Geometry: final body of the model. Coordinates: model frame, mm. A direction names the side the tool comes from. Give positions to 0.01 mm unless a question says otherwise; leave off trailing zeros. Write each loop counter-clockwise with the first axis right and the second up, starting at its lowest first coordinate (ties: lowest second). Pieces come first, ordered by that corner, then holes.
from build123d import *

# Parameters (mm, degrees)
F1_DEPTH = 580
F2_R     = 6.25
F3_DEPTH = 80.001


with BuildPart() as f1:
    # F0 (on Front) → F1 (new body, symmetric)
    with BuildSketch(Plane.XZ):
        with BuildLine():
            ThreePointArc((40, 30), (37.071068, 37.071068), (30, 40))
            Line((30, 40), (-30, 40))
            ThreePointArc((-30, 40), (-37.071068, 37.071068), (-40, 30))
            Line((-40, 30), (-40, -30))
            ThreePointArc((-40, -30), (-37.071068, -37.071068), (-30, -40))
            Line((-30, -40), (30, -40))
            ThreePointArc((30, -40), (37.071068, -37.071068), (40, -30))
            Line((40, -30), (40, 30))
        make_face()
        with BuildLine():
            ThreePointArc((30, 35), (33.535534, 33.535534), (35, 30))
            Line((35, 30), (35, -30))
            ThreePointArc((35, -30), (33.535534, -33.535534), (30, -35))
            Line((30, -35), (-30, -35))
            ThreePointArc((-30, -35), (-33.535534, -33.535534), (-35, -30))
            Line((-35, -30), (-35, 30))
            ThreePointArc((-35, 30), (-33.535534, 33.535534), (-30, 35))
            Line((-30, 35), (30, 35))
        make_face(mode=Mode.SUBTRACT)
    extrude(amount=F1_DEPTH, both=True)

    # F2 (on face) → F3 (cut, through all)
    with BuildSketch(Plane.YZ.offset(40)):
        with Locations((-539, 0)):
            Circle(F2_R)
        with Locations((539, 0)):
            Circle(F2_R)
    extrude(amount=-F3_DEPTH, mode=Mode.SUBTRACT)


solid = f1.part
Q1. Access query for faces 1 (the flat face through (0, -8, 40)), 2 (the flat face through (-35, -8, 0)). Directions: +Z, -Z, +X, -X, +Y, -Y. A direction counts if a zero-diameter tool reaches every point of the face in a straight line with its end or side. Return the directions, or none.
Filled sheet:
face 1: +Z, +X, -X, +Y, -Y
face 2: +Y, -Y
Q2. Section A-A on z = -20.5. Output: boundary loops of the cut face in (x, y).
Filled sheet:
outline: (-40, -580) - (-35, -580) - (-35, 580) - (-40, 580) - close; (35, -580) - (40, -580) - (40, 580) - (35, 580) - close
Q3. Section B-B on x = -0.5. Output: boundary loops of the cut face in (y, z), plus the area to 3 significant figures.
Filled sheet:
outline: (-580, -40) - (580, -40) - (580, -35) - (-580, -35) - close; (-580, 35) - (580, 35) - (580, 40) - (-580, 40) - close
area: 11,600 mm2
Q4. Section C-C on y = 92.5. Output: boundary loops of the cut face in (x, z), plus the area to 3 significant figures.
Filled sheet:
outline: (-40, -30) arc R10 ccw to (-30, -40) - (30, -40) arc R10 ccw to (40, -30) - (40, 30) arc R10 ccw to (30, 40) - (-30, 40) arc R10 ccw to (-40, 30) - close; hole (-35, -30) arc R5 ccw to (-30, -35) - (30, -35) arc R5 ccw to (35, -30) - (35, 30) arc R5 ccw to (30, 35) - (-30, 35) arc R5 ccw to (-35, 30) - close
area: 1,440 mm2
Q5. Ray query, line 1 along Z through (x, y) = (-6, 95); line 2 along Z through (x, y) = (38.55, -539). Return the intervals inside material, ascending.
Filled sheet:
line 1: z = -40 to -35, 35 to 40
line 2: z = -35.19 to -6.25, 6.25 to 35.19
Q6. Pin query (flat end, axial travel): P1, Ø12, axis at x = -25, z = 24.5, coming from the +Y side. Return the tip coordinate at first contact, or that it passes through.
Filled sheet:
P1: passes through
Q7. Pull-direction query (Z, two-part tool) for faces 3 (the flat face through (-0.2, 580, -35.4)), 4 (the flat face through (0, -8, -40)), 5 (the flat face through (0, -8, -35)); classes: released by +Z, released by -Z, zero draft, split by the parting line, or undercut.
Filled sheet:
face 3: zero draft
face 4: released by -Z
face 5: undercut
